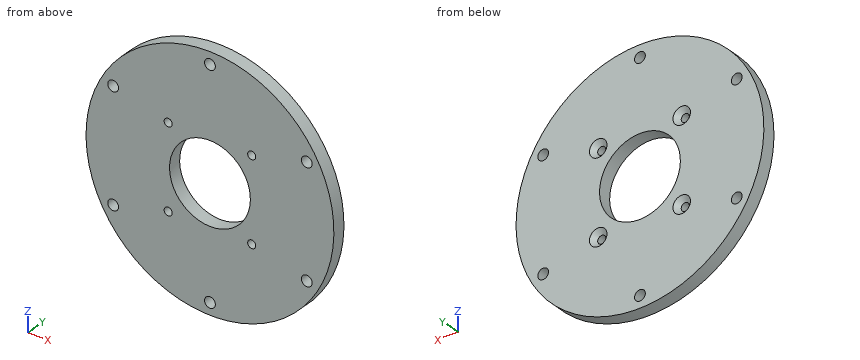
```python
from build123d import *

# Parameters (mm, degrees)
SKETCH1_R                                            = 46
SKETCH1_R_2                                          = 19.25
SKETCH1_R_3                                          = 1.5
BOSS_EXTRUDE1_DEPTH                                  = 5
SKETCH3_R                                            = 2
CUT_EXTRUDE2_DEPTH                                   = 66.245689513
SKETCH7_R                                            = 15
CUT_EXTRUDE3_DEPTH                                   = 66.245689513
CSK_FOR_M3_SOCKET_COUNTERSUNK_HEAD_SCREW_D           = 2.8
CSK_FOR_M3_SOCKET_COUNTERSUNK_HEAD_SCREW_CSINK_D     = 6.5
CSK_FOR_M3_SOCKET_COUNTERSUNK_HEAD_SCREW_CSINK_ANGLE = 90


with BuildPart() as part:
    # Sketch1 → Boss-Extrude1 (new body)
    # profile 1 of 2: a face of its own
    with BuildSketch(Plane(origin=(0, 0, 0), x_dir=(1, 0, 0), z_dir=(0, 1, 0))):
        with Locations(Location((0, 0, 0), (0, 0, 270))):
            Circle(SKETCH1_R)
        Circle(SKETCH1_R_2, mode=Mode.SUBTRACT)
        with Locations(Location((-15.5, -15.5, 0), (0, 0, 270))):
            Circle(SKETCH1_R_3, mode=Mode.SUBTRACT)
        with Locations(Location((15.5, -15.5, 0), (0, 0, 270))):
            Circle(SKETCH1_R_3, mode=Mode.SUBTRACT)
        with Locations(Location((15.5, 15.5, 0), (0, 0, 270))):
            Circle(SKETCH1_R_3, mode=Mode.SUBTRACT)
        with Locations(Location((-15.5, 15.5, 0), (0, 0, 270))):
            Circle(SKETCH1_R_3, mode=Mode.SUBTRACT)
    # profile 2 of 2: a face of its own
    with BuildSketch(Plane(origin=(0, 0, 0), x_dir=(1, 0, 0), z_dir=(0, 1, 0))):
        Circle(SKETCH1_R_2)
    extrude(amount=BOSS_EXTRUDE1_DEPTH)

    # Sketch3 → Cut-Extrude2 (cut, through all)
    with BuildSketch(Plane.XZ):
        with Locations(Location((0, 41.5, 0), (0, 0, 270))):
            Circle(SKETCH3_R)
        with Locations(Location((35.940054257, 20.75, 0), (0, 0, 270))):
            Circle(SKETCH3_R)
        with Locations(Location((35.940054257, -20.75, 0), (0, 0, 270))):
            Circle(SKETCH3_R)
        with Locations(Location((0, -41.5, 0), (0, 0, 270))):
            Circle(SKETCH3_R)
        with Locations(Location((-35.940054257, -20.75, 0), (0, 0, 270))):
            Circle(SKETCH3_R)
        with Locations(Location((-35.940054257, 20.75, 0), (0, 0, 270))):
            Circle(SKETCH3_R)
    extrude(amount=-CUT_EXTRUDE2_DEPTH, mode=Mode.SUBTRACT)

    # Sketch7 → Cut-Extrude3 (cut, through all)
    with BuildSketch(Plane.XZ):
        with Locations(Location((0, 0, 0), (0, 0, 270))):
            Circle(SKETCH7_R)
    extrude(amount=-CUT_EXTRUDE3_DEPTH, mode=Mode.SUBTRACT)

    # CSK for M3 socket countersunk head screw (through all)
    with Locations(Plane(origin=(15.5, 5, -15.5), x_dir=(0, 0, 1), z_dir=(0, 1, 0))):
        with Locations((0, 0), (31, 0), (31, -31), (0, -31)):
            CounterSinkHole(CSK_FOR_M3_SOCKET_COUNTERSUNK_HEAD_SCREW_D / 2, CSK_FOR_M3_SOCKET_COUNTERSUNK_HEAD_SCREW_CSINK_D / 2, counter_sink_angle=CSK_FOR_M3_SOCKET_COUNTERSUNK_HEAD_SCREW_CSINK_ANGLE)


solid = part.part
```
Work out the finished part from the listing and answer in its coordinate system (mm). Round coordinates to 2 decimals unless told otherwise and drop trailing zeros. Write each loop counter-clockwise with the first axis right and the second up, starting at its lowest first coordinate (ties: lowest second). Pieces come first, ordered by that corner, then holes. Notation, with made-up numbers: (-29.5, 80) - (20.5, 80) arc R25 cw to (20.5, 118) - close; hole circle Ø11 at (41, 48). An arc over 180 degrees is marked (long way). Return JSON: item names as keys, results as strings. Group by question number.
Q1. The part is cut by section D-D on y = 2. Count the separate pieces of the cut face and the enclosed holes in it, then the cut area to 3 significant figures.
Q2. Find the intervals of material crossed by L1, parallel to Z at x = 15.5, y = 1.6; L2, parallel to Z at x = 6.5, y = 3.8; L3, parallel to Z at x = 5, y = 0.55, in increasing order.
Q3. The part is cut by section A-A on x = 0. Write down the section's boundary in (y, z), then the cut area to 3 significant figures.
Q4. The part is cut by section C-C on x = -10.5. Write down the section's boundary in (y, z).
Q5. Each of these flat-tipped pins is pushed along its axis until it touches: pin 1 Ø3.5 at (x, z) = (-15.5, 15.5) entering from -Y; pin 2 Ø3 at (x, z) = (-35.94, 20.75) entering from +Y; pin 3 Ø1 at (x, y) = (-4, 3) entering from -Z; pin 4 Ø4 at (x, z) = (15.5, 15.5) entering from +Y. Where does it stop, or does it pass through?
Q6. The part is cut by section B-B on z = -41.5. Write down the section's boundary in (x, y), then the cut area to 3 significant figures.
Solved:
{
 "1": {"separate pieces": "1", "enclosed holes": "11", "area": "5,840 mm²"},
 "2": {"L1": "-43.31 to -17, -14 to 14, 17 to 43.31", "L2": "-45.54 to -13.52, 13.52 to 45.54", "L3": "-45.73 to -14.14, 14.14 to 45.73"},
 "3": {"outline": "(0, -46) - (5, -46) - (5, -43.5) - (0, -43.5) - close; (0, -39.5) - (5, -39.5) - (5, -15) - (0, -15) - close; (0, 15) - (5, 15) - (5, 39.5) - (0, 39.5) - close; (0, 43.5) - (5, 43.5) - (5, 46) - (0, 46) - close", "area": "270 mm²"},
 "4": {"outline": "(0, -44.79) - (5, -44.79) - (5, -10.71) - (0, -10.71) - close; (0, 10.71) - (5, 10.71) - (5, 44.79) - (0, 44.79) - close"},
 "5": {"pin 1": "y = 0", "pin 2": "through", "pin 3": "z = -45.87", "pin 4": "y = 3.75"},
 "6": {"outline": "(-19.84, 0) - (-2, 0) - (-2, 5) - (-19.84, 5) - close; (2, 0) - (19.84, 0) - (19.84, 5) - (2, 5) - close", "area": "178 mm²"}
}
